Source: CAD feature listing. Evaluate the final solid. Frame: model axes, mm. Coordinates: 2 decimals unless noted, no trailing zeros. Order: outer loops, then holes, each group sorted by start corner. A loop starts at its lowest first (then second) coordinate and runs counter-clockwise, first axis right, second up.
```python
from build123d import *

# Parameters (mm, degrees)
SKETCH1_W           = 50
SKETCH1_H           = 10
BOSS_EXTRUDE1_DEPTH = 5


with BuildPart() as part:
    # Sketch1 → Boss-Extrude1 (new body)
    with BuildSketch(Plane(origin=(0, 0, 0), x_dir=(1, 0, 0), z_dir=(0, 1, 0))):
        Polygon((-12.5, 12.5), (12.5, 12.5), (12.5, 17.5), (32.5, 17.5), (32.5, 12.5), (47.5, 12.5), (47.5, 5.5), (42.5, 5.5), (42.5, -5.5), (47.5, -5.5), (47.5, -12.5), (32.5, -12.5), (32.5, -17.5), (12.5, -17.5), (12.5, -12.5), (-12.5, -12.5), (-12.5, -17.5), (-32.5, -17.5), (-32.5, -12.5), (-47.5, -12.5), (-47.5, -5.5), (-42.5, -5.5), (-42.5, 5.5), (-47.5, 5.5), (-47.5, 12.5), (-32.5, 12.5), (-32.5, 17.5), (-12.5, 17.5), align=None)
        Rectangle(SKETCH1_W, SKETCH1_H, mode=Mode.SUBTRACT)
    extrude(amount=BOSS_EXTRUDE1_DEPTH)


solid = part.part
```
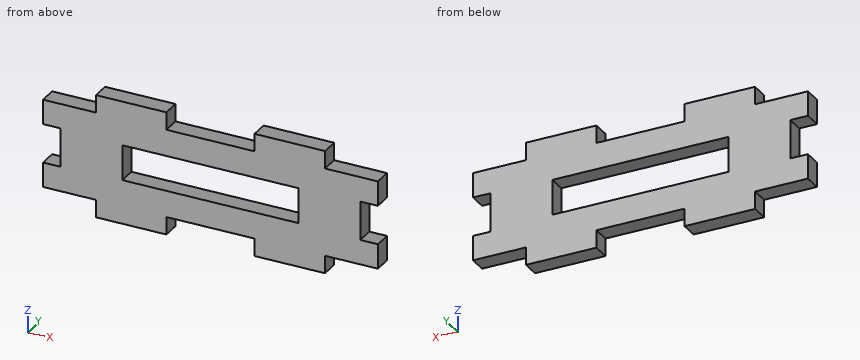
Q1. Section query A-A on z = 3. Output: boundary loops of the cut face in (x, y), plus the area to 3 significant figures.
Solutions:
outline: (-42.5, 0) - (-25, 0) - (-25, 5) - (-42.5, 5) - close; (25, 0) - (42.5, 0) - (42.5, 5) - (25, 5) - close
area: 175 mm2
Q2. Pin query (flat end, axial travel): P1, Ø2.5, axis at x = -38, y = 3, coming from the +Z side; P2, Ø2.5, axis at y = 2, z = 2, coming from the +X side; P3, Ø1.5, axis at y = 3.5, z = -15, coming from the +X side. Return the tip coordinate at first contact, or that it passes through.
Solutions:
P1: stops at z = 12.5
P2: stops at x = 42.5
P3: stops at x = 32.5
Q3. Section query D-D on x = 40.5. Output: boundary loops of the cut face in (y, z).
Solutions:
outline: (0, -12.5) - (5, -12.5) - (5, 12.5) - (0, 12.5) - close
Q4. Material intervals for line 1 along Z through (x, y) = (3, 4.35); line 2 along Z through (x, y) = (-16, 1.7); line 3 along X through (y, z) = (2.85, -1), sorted ascending.
Solutions:
line 1: z = -12.5 to -5, 5 to 12.5
line 2: z = -17.5 to -5, 5 to 17.5
line 3: x = -42.5 to -25, 25 to 42.5
Q5. Section query B-B on x = -18.5. Output: boundary loops of the cut face in (y, z).
Solutions:
outline: (0, -17.5) - (5, -17.5) - (5, -5) - (0, -5) - close; (0, 5) - (5, 5) - (5, 17.5) - (0, 17.5) - close
